Build history of the part. All positions in model axes, mm. A direction names the side the tool comes from. Coordinates: 2 decimals unless noted, no trailing zeros. Order: outer loops, then holes, each group sorted by start corner. A loop starts at its lowest first (then second) coordinate and runs counter-clockwise, first axis right, second up. Notation, with made-up numbers: M 56,37 L 102,37 A28 ccw 102,59 Z; hole C -17,-17 d8. An arc over 180 degrees is marked long. Write item = value, one per line. Start each with the question number.
Q1. Pull direction Y, two halves, no side cores. Call faces 1 (the face through (-0.5, 10, -0.2)), 2 (the face through (-10, 0.5, -0.2)), 3 (the face through (-0.51, 7.47, -8.73)): released by +Y, released by -Y, zero draft, split by the parting line, or undercut.
Q2. Band-saw the part on A-A on z = 10. Write the cut outline in (x, y), plus the area to 3 significant figures.
Q3. Band-saw the part on B-B on x = -6.5. Write the cut outline in (y, z).
Q4. 3-axis set-ups, long thin cutter, end or side, ignore diameter. For faces 4 (the face through (-2.8, 0.6, 15)), 5 (the face through (-4, 1, 0)): which of +Z, -Z, +X, -X, +Y, -Y reach the whole face in a straight line?
Q5. Band-saw the part on D-D on z = 1.5. Write the cut outline in (x, y), plus the area to 3 significant figures.
Q6. Drill centre lines: probe 1 along Z at (x, y) = (-0.15, 6.5); probe 2 along Y at (x, z) = (-0.15, 10); probe 3 along X at (y, z) = (0.7, 0). Where is each one in solid material? Low to high.
Q7. Band-saw the part on C-C on y = 7.5. Write the cut outline in (x, z), plus the area to 3 significant figures.
Q8. Pin check, flat tips, straight feed: P1, Ø1.5, axis at x = -7.5, z = -5.5, coming from the +Y side; P2, Ø2, axis at x = -6.5, z = 0, coming from the +Y side; P3, Ø2.5, axis at y = 5.5, z = 7, coming from the -X side. Stop position of each tip, or through.
Autodesk Inventor part; units mm, degrees
ref_plane "YZ Plane" through (0, 0, 0) normal (1, 0, 0) x (0, 1, 0)
ref_plane "XZ Plane" through (0, 0, 0) normal (0, 1, 0) x (-1, 0, 0)
ref_plane "XY Plane" through (0, 0, 0) normal (0, 0, 1) x (1, 0, 0)
sketch "Náčrt1" plane through (0, 0, 0) normal (0, 0, 1) x (1, 0, 0)
  line L0 (-10, 0) -> (0, 0)
  line L1 (0, 0) -> (0, 10)
  line L2 (0, 10) -> (-1, 10)
  line L3 (-1, 10) -> (-1, 1)
  line L4 (-1, 1) -> (-10, 1)
  line L5 (-10, 1) -> (-10, 0)
  line L6 (0, 12) -> (0, -2)
  line L7 (-12, 0) -> (2, 0)
  point P0 (0, 0)
  dimension "d0" = 10
  dimension "d1" = 10
  dimension "d2" = 1
  dimension "d3" = 1
extrude "Vysunutí1" add sketch "Náčrt1" along normal mid plane 30
sketch "Náčrt2" plane through (0, 0, 15) normal (1, 0, 0) x (0, 0, -1)
  line L0 (30, 10) -> (0, 10)
  line L1 (30, 10) -> (30, 0)
  point P0 (15, 0)
  point P1 (5, 6.5)
  point P2 (25, 6.5)
  point P3 (30, 5)
  dimension "d6" = 3.5
  dimension "d7" = 3.5
  dimension "d8" = 20
  dimension "d9" = 5
hole "Díra1" at (0, 6.5, 10) at (0, 6.5, -10) direction (-1, 0, 0) diameter 3.2 end through all
sketch "Náčrt3" plane through (-10, 1, 15) normal (0, 1, 0) x (1, 0, 0)
  line L0 (0, 0) -> (0, 30)
  line L1 (0, 0) -> (0, 30)
  line L2 (9, 0) -> (0, 0)
  line L3 (9, 30) -> (9, 0)
  line L4 (0, 30) -> (9, 30)
  point P0 (10, 15)
  point P1 (3.5, 15)
  dimension "d17" = 3.5
  dimension "d18" = 15
hole "Díra2" at (-6.5, 1, 0) direction (0, -1, 0) diameter 2.459 end through all
properties part number "y_cable_adaptor_holder" material "Hliník 6061"
Recorded:
q1.face_1 = released by +Y
q1.face_2 = zero draft
q1.face_3 = undercut
q2.outline = M -10,0 L 0,0 L 0,4.9 L -1,4.9 L -1,1 L -10,1 Z; M -1,8.1 L 0,8.1 L 0,10 L -1,10 Z
q2.area = 15.8 mm2
q3.outline = M 0,-15 L 1,-15 L 1,-1.23 L 0,-1.23 Z; M 0,1.23 L 1,1.23 L 1,15 L 0,15 Z
q4.face_4 = +Z, +X, -X, +Y, -Y
q4.face_5 = +Z, -Z, -X, +Y
q5.outline = M -10,0 L 0,0 L 0,10 L -1,10 L -1,1 L -10,1 Z
q5.area = 19.0 mm2
q6.probe_1 = -15 to -11.6, -8.4 to 8.4, 11.6 to 15
q6.probe_2 = 0 to 4.9, 8.1 to 10
q6.probe_3 = -10 to -7.73, -5.27 to 0
q7.outline = M -1,-15 L 0,-15 L 0,-11.25 L -1,-11.25 Z; M -1,-8.75 L 0,-8.75 L 0,8.75 L -1,8.75 Z; M -1,11.25 L 0,11.25 L 0,15 L -1,15 Z
q7.area = 25.0 mm2
q8.P1 = 1
q8.P2 = through
q8.P3 = -1
